Geometry: final body of the model. Coordinates: model frame, mm. A direction names the side the tool comes from. Give positions to 0.01 mm unless a question says otherwise; leave off trailing zeros. Write each loop counter-clockwise with the first axis right and the second up, starting at its lowest first coordinate (ties: lowest second). Pieces come first, ordered by that corner, then holes. Notation, with made-up numbers: M 37.5,-26.5 L 75.5,-26.5 A20 ccw 75.5,10.5 Z; hole C 60,-24.5 d1. An arc over 180 degrees is marked long. Answer as a JSON object with one key per item and string values.
from build123d import *

# Parameters (mm, degrees)
SKETCH1_W                         = 2
SKETCH1_H                         = 100
F_1_2_20_TAPPED_HOLE1_D           = 11.50874
F_1_2_20_TAPPED_HOLE1_DEPTH       = 30
F_1_2_20_TAPPED_HOLE1_CSINK_D     = 13.97
F_1_2_20_TAPPED_HOLE1_CSINK_ANGLE = 90
F_1_2_20_TAPPED_HOLE1_TIP         = 3.45757432


with BuildPart() as part:
    # Sketch1 → Revolve1 (revolve)
    with BuildSketch(Plane.XY):
        Polygon((0, 58), (0, 0), (21.5, 0), (21.5, 38.666666667), (15, 58), (2, 58), align=None)
        with Locations((1, 108)):
            Rectangle(SKETCH1_W, SKETCH1_H)
    revolve(axis=Axis((0, 0, 0), (0, 1, 0)))

    # 1/2-20 Tapped Hole1
    with Locations(Plane(origin=(0, 0, 0), x_dir=(-1, 0, 0), z_dir=(0, -1, 0))):
        with Locations((0, 0)):
            CounterSinkHole(F_1_2_20_TAPPED_HOLE1_D / 2, F_1_2_20_TAPPED_HOLE1_CSINK_D / 2, depth=F_1_2_20_TAPPED_HOLE1_DEPTH, counter_sink_angle=F_1_2_20_TAPPED_HOLE1_CSINK_ANGLE)
            with Locations((0, 0, -(F_1_2_20_TAPPED_HOLE1_DEPTH + F_1_2_20_TAPPED_HOLE1_TIP / 2))):  # 118° drill point
                Cone(0, F_1_2_20_TAPPED_HOLE1_D / 2, F_1_2_20_TAPPED_HOLE1_TIP, mode=Mode.SUBTRACT)


solid = part.part
1) Line query: line 1 (Z direction, x = 0, y = 24); line 2 (Y direction, x = 2.5, z = -10.5); line 3 (X direction, y = 66.5, z = 1.5). Output: solid intervals per line, ascending. Write a range as from..to.
Geometry check:
{"line 1": "z = -21.5..-5.75, 5.75..21.5", "line 2": "y = 0..58", "line 3": "x = -1.32..1.32"}
2) Cut plane B-B on y = 11. Return loops of the section in (x, z).
Geometry check:
{"outline": "C 0,0 d43; hole C 0,0 d11.51"}
3) Pull-direction query (X, two-part tool) for faces 1 (the cylindrical face through (-2.799, 19.604, -21.317)), 2 (the conical face through (0.217, 32.857, 0.976)), 3 (the flat face through (0, 58, 3)), 4 (the cylindrical face through (-0.749, 15.817, -5.705)); classes: pulls with the +X half, pulls with the -X half, needs draft (parallel to the pull), parting line crosses it, or undercut.
Geometry check:
{"face 1": "parting line crosses it", "face 2": "undercut", "face 3": "needs draft", "face 4": "undercut"}
4) Cut plane A-A on y = 105. Return loops of the section in (x, z), and give its area (3 significant figures).
Geometry check:
{"outline": "C 0,0 d4", "area": "12.6 mm2"}
5) Set-up query: faces 5 (the flat face through (5.1, 0, -5.1)), 6 (the cylindrical face through (0, 109, 2)). Return all of +Z, -Z, +X, -X, +Y, -Y with unobstructed straight access to the full face (end or side cutting, diameter ignored); none if empty.
Geometry check:
{"face 5": "+Z, -Z, +X, -X, -Y", "face 6": "+Y"}
6) Contact query for flat-ended pins moving along their axis: P1, Ø12, axis at x = 9, y = 70.5, coming from the -Z side; P2, Ø2, axis at x = -7.5, z = -1, coming from the +Y side; P3, Ø1, axis at y = 51.5, z = 10, coming from the +X side; P4, Ø2, axis at x = 0, y = 62, coming from the +Z side. Output: stop coordinate, or through.
Geometry check:
{"P1": "passes through", "P2": "stops at y = 58", "P3": "stops at x = 14.38", "P4": "stops at z = 2"}
